Geometry check sheet. Reference: the model listing, model coordinates, mm. Face numbers are marked on the shaded views. A direction names the side the tool comes from. Round coordinates to 2 decimals unless told otherwise and drop trailing zeros. Write each loop counter-clockwise with the first axis right and the second up, starting at its lowest first coordinate (ties: lowest second). Pieces come first, ordered by that corner, then holes. Notation, with made-up numbers: (0.5, 52) -> (58.5, 52) arc R11 ccw to (58.5, 72) -> close; hole circle Ø3 at (8, 88.25). An arc over 180 degrees is marked (long way). Use a Markdown table: item, result.
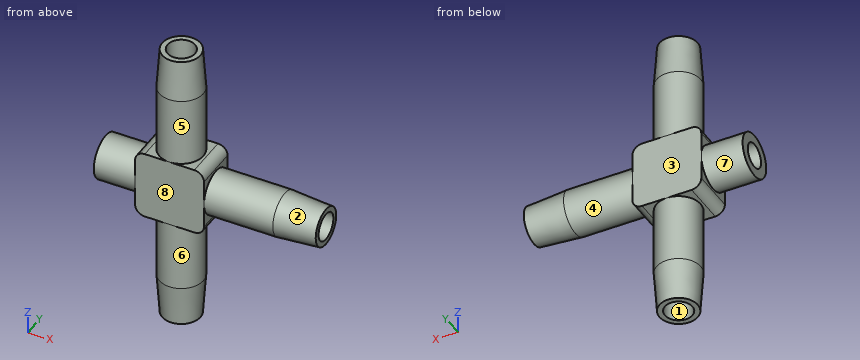
```python
from build123d import *

# Parameters (mm, degrees)
SKETCH1_W               = 10
SKETCH1_H               = 10
BOSS_EXTRUDE1_DEPTH     = 6.4
SKETCH2_R               = 3.2
BOSS_EXTRUDE2_DEPTH     = 10
SKETCH4_R               = 3.2
BOSS_EXTRUDE3_DEPTH     = 10
SKETCH8_R               = 3.2
BOSS_EXTRUDE4_DEPTH     = 6
BOSS_EXTRUDE4_TAPER     = 4
SKETCH10_R              = 3.2
BOSS_EXTRUDE5_DEPTH     = 6
BOSS_EXTRUDE5_TAPER     = 4
FILLET1_R               = 1.4
SKETCH11_R              = 2
CUT_EXTRUDE5_DEPTH      = 48.391560488
CUT_EXTRUDE6_REACH      = 36.029
CUT_EXTRUDE6_END_RADIUS = 2
SKETCH9_R               = 2
BOSS_EXTRUDE6_START     = 6
SKETCH12_R              = 3.2
SKETCH12_R_2            = 1.8
BOSS_EXTRUDE6_DEPTH     = 6


with BuildPart() as part:
    # Sketch1 → Boss-Extrude1 (new body)
    with BuildSketch(Plane(origin=(0, 0, 0), x_dir=(1, 0, 0), z_dir=(0, 1, 0))):
        Rectangle(SKETCH1_W, SKETCH1_H)
    extrude(amount=BOSS_EXTRUDE1_DEPTH)

    # Sketch2 → Boss-Extrude2 (add)
    with BuildSketch(Plane.XY.offset(5)):
        with Locations(Location((0, 3.2, 0), (0, 0, 270))):
            Circle(SKETCH2_R)
    boss_extrude2 = extrude(amount=BOSS_EXTRUDE2_DEPTH)

    # Sketch4 → Boss-Extrude3 (add)
    with BuildSketch(Plane(origin=(5, 0, 0), x_dir=(0, 0, -1), z_dir=(1, 0, 0))):
        with Locations(Location((0, 3.2, 0), (0, 0, 270))):
            Circle(SKETCH4_R)
    extrude(amount=BOSS_EXTRUDE3_DEPTH)

    # Sketch8 → Boss-Extrude4 (add)
    with BuildSketch(Plane(origin=(15, 0, 0), x_dir=(0, 0, -1), z_dir=(1, 0, 0))):
        with Locations(Location((0, 3.2, 0), (0, 0, 270))):
            Circle(SKETCH8_R)
    extrude(amount=BOSS_EXTRUDE4_DEPTH, taper=BOSS_EXTRUDE4_TAPER)

    # Sketch10 → Boss-Extrude5 (add)
    with BuildSketch(Plane.XY.offset(15)):
        with Locations(Location((0, 3.2, 0), (0, 0, 270))):
            Circle(SKETCH10_R)
    boss_extrude5 = extrude(amount=BOSS_EXTRUDE5_DEPTH, taper=BOSS_EXTRUDE5_TAPER)

    # Mirror2: Boss-Extrude2, Boss-Extrude5 across plane
    add(boss_extrude2.mirror(Plane.XY))
    add(boss_extrude5.mirror(Plane.XY))

    # Fillet1
    fillet1_edges = [part.edges().sort_by_distance(p)[0] for p in [
        (-5, 3.2, -5),
        (5, 3.2, -5),
        (5, 3.2, 5),
        (-5, 3.2, 5),
    ]]
    fillet(fillet1_edges, radius=FILLET1_R)

    # Sketch11 → Cut-Extrude5 (cut, through all)
    with BuildSketch(Plane.XY.offset(21)):
        with Locations((0, 3.2)):
            Circle(SKETCH11_R)
    extrude(amount=-CUT_EXTRUDE5_DEPTH, mode=Mode.SUBTRACT)

    # Cut-Extrude6: up to this cylinder (the profile starts outside it)
    cut_extrude6_end = Plane(origin=(0, 3.2, 0), z_dir=(0, 0, 1)) * Cylinder(CUT_EXTRUDE6_END_RADIUS, 77.058, mode=Mode.PRIVATE)
    # Sketch9 → Cut-Extrude6 (cut, up to the surface)
    with BuildSketch(Plane(origin=(21, 0, 0), x_dir=(0, 0, -1), z_dir=(1, 0, 0)), mode=Mode.PRIVATE) as cut_extrude6_sk1:
        with Locations((0, 3.2)):
            Circle(SKETCH9_R)
    cut_extrude6_tool1 = extrude(cut_extrude6_sk1.sketch, amount=-CUT_EXTRUDE6_REACH, mode=Mode.PRIVATE) - cut_extrude6_end
    add(cut_extrude6_tool1.solids().sort_by_distance((21, 3.2, 0))[0], mode=Mode.SUBTRACT)

    # Sketch12 → Boss-Extrude6 (add)
    with BuildSketch(Plane.ZY.offset(5).offset(BOSS_EXTRUDE6_START)):
        with Locations(Location((0, 3.2, 0), (0, 0, 270))):
            Circle(SKETCH12_R)
        with Locations((0, 3.2)):
            Circle(SKETCH12_R_2, mode=Mode.SUBTRACT)
    extrude(amount=-BOSS_EXTRUDE6_DEPTH)


solid = part.part
```
(1) Section check B-B on x = 5.5. Record the cut outline in (y, z), plus the area to 3 significant figures.
A:
| item | result |
|---|---|
| outline | circle Ø6.4 at (3.2, 0); hole circle Ø4 at (3.2, 0) |
| area | 19.6 mm2 |
(2) Release check for a two-part mould opening along Y. For the marked faces 1, 2 and 3 record: +Y half, -Y half, draft (parallel to the pull), parting line (faces both ways), or undercut.
A:
| item | result |
|---|---|
| face 1 | undercut |
| face 2 | parting line |
| face 3 | +Y half |
(3) Thickness scan on line 1 (Y direction, x = 0, z = -3); line 2 (Z direction, x = 13, y = 3); line 3 (Y direction, x = 0.5, z = -17). Record the ranges inside material, lowest first.
A:
| item | result |
|---|---|
| line 1 | y = 0 to 1.2, 5.2 to 6.4 |
| line 2 | z = -3.19 to -1.99, 1.99 to 3.19 |
| line 3 | y = 0.18 to 1.26, 5.14 to 6.22 |
(4) Section check C-C on y = 3.2. State how many separate pieces and enclosed holes the cut face has, plus the area to 3 significant figures.
A:
| item | result |
|---|---|
| separate pieces | 3 |
| enclosed holes | 0 |
| area | 171 mm2 |
(5) Section check A-A on z = 11. Record the cut outline in (x, y), plus the area to 3 significant figures.
A:
| item | result |
|---|---|
| outline | circle Ø6.4 at (0, 3.2); hole circle Ø4 at (0, 3.2) |
| area | 19.6 mm2 |
(6) Gauge pin test, flat ends, axial feed: pin 1 Ø10 at (x, z) = (14.5, 2.5) entering from +Y; pin 2 Ø3.5 at (y, z) = (3.2, 0) entering from +X; pin 3 Ø2 at (y, z) = (3.2, 0) entering from +X. Record the tip position at first contact, or that the pin passes through.
A:
| item | result |
|---|---|
| pin 1 | stops at y = 6.4 |
| pin 2 | stops at x = -0.97 |
| pin 3 | stops at x = -1.73 |
(7) Access from +Z, -Z, +X, -X, +Y, -Y to the whole of each face (thin tool, end or side, straight path). Record for the marked faces 4, 5, 6, 7 and 8.
A:
| item | result |
|---|---|
| face 4 | +X |
| face 5 | +Z |
| face 6 | -Z |
| face 7 | -X |
| face 8 | +Z, -Z, +X, -X, -Y |
